```python
from build123d import *

# Parameters (mm, degrees)
EXTRUDE_1_DEPTH       = 245
EXTRUDE_3_DEPTH       = 245
PATTERN_CURVE_1_COUNT = 19
PATTERN_CURVE_1_PITCH = 9.75
SKETCH_3_R            = 2.05
CUT_EXTRUDE_1_DEPTH   = 10
CUT_EXTRUDE_START     = -10
SKETCH_5_R            = 2.05
CUT_EXTRUDE_2_DEPTH   = 10
SKETCH_6_R            = 2.5
CUT_EXTRUDE_3_DEPTH   = 8
SKETCH_7_R            = 2.6
CUT_EXTRUDE_4_DEPTH   = 6
SKETCH_8_R            = 3.4
SKETCH_8_R_2          = 4.5
CUT_EXTRUDE_5_DEPTH   = 6
CUT_EXTRUDE_START_2   = -8
SKETCH_10_R           = 2.5
CUT_EXTRUDE_7_DEPTH   = 8
SKETCH_12_R           = 1.3
SKETCH_12_R_2         = 1.6
SKETCH_12_R_3         = 2.1
CUT_EXTRUDE_8_DEPTH   = 8


with BuildPart() as part:
    # Эскиз1 → Вытянуть1 (new body)
    with BuildSketch(Plane.XY):
        with BuildLine():
            Line((0, 45), (2.564446908, 45))
            ThreePointArc((2.564446908, 45), (3.247630994, 44.730246195), (3.562232066, 44.066519011))
            Line((3.562232066, 44.066519011), (5.5, 15))
            Line((5.5, 15), (194.5, 15))
            Line((194.5, 15), (196.437767934, 44.066519011))
            ThreePointArc((196.437767934, 44.066519011), (196.752369006, 44.730246195), (197.435553092, 45))
            Line((197.435553092, 45), (200, 45))
            Line((200, 45), (200, 0))
            Line((200, 0), (0, 0))
            Line((0, 0), (0, 45))
        make_face()
    extrude(amount=EXTRUDE_1_DEPTH)

    # Эскиз2 → Вытянуть3 (add)
    with BuildSketch(Plane.XY.offset(245)):
        with BuildLine():
            Line((11.5, 44.5), (10, 15))
            Line((10, 15), (14, 15))
            Line((14, 15), (12.5, 44.5))
            ThreePointArc((12.5, 44.5), (12, 45), (11.5, 44.5))
        make_face()
    extrude_3 = extrude(amount=-EXTRUDE_3_DEPTH)

    # Кривая1: Вытянуть3 ×19
    with Locations(*[(i * PATTERN_CURVE_1_PITCH, 0, 0) for i in range(1, PATTERN_CURVE_1_COUNT)]):
        add(extrude_3)

    # Эскиз3 → Вырез-Вытянуть1 (cut)
    with BuildSketch(Plane.XY.offset(245)):
        with Locations((20, 5)):
            Circle(SKETCH_3_R)
        with Locations((100, 5)):
            Circle(SKETCH_3_R)
        with Locations((180, 5)):
            Circle(SKETCH_3_R)
    extrude(amount=-CUT_EXTRUDE_1_DEPTH, mode=Mode.SUBTRACT)

    # Эскиз5 → Вырез-Вытянуть2 (cut)
    with BuildSketch(Plane(origin=(0, 0, 0), x_dir=(-1, 0, 0), z_dir=(0, 0, -1)).offset(CUT_EXTRUDE_START)):
        with Locations(Location((-180, 5, 0), (0, 0, 180))):
            Circle(SKETCH_5_R)
        with Locations(Location((-100, 5, 0), (0, 0, 180))):
            Circle(SKETCH_5_R)
        with Locations(Location((-20, 5, 0), (0, 0, 180))):
            Circle(SKETCH_5_R)
    extrude(amount=CUT_EXTRUDE_2_DEPTH, mode=Mode.SUBTRACT)

    # Эскиз6 → Вырез-Вытянуть3 (cut)
    with BuildSketch(Plane(origin=(0, 0, 0), x_dir=(-1, 0, 0), z_dir=(0, 0, -1))):
        with Locations((-4, 6)):
            Circle(SKETCH_6_R)
        with Locations(Location((-196, 6, 0), (0, 0, 180))):
            Circle(SKETCH_6_R)
    extrude(amount=-CUT_EXTRUDE_3_DEPTH, mode=Mode.SUBTRACT)

    # Эскиз7 → Вырез-Вытянуть4 (cut)
    with BuildSketch(Plane.ZY):
        with Locations(Location((22.5, 20, 0), (0, 0, 270))):
            Circle(SKETCH_7_R)
        with Locations(Location((222.5, 20, 0), (0, 0, 270))):
            Circle(SKETCH_7_R)
        with Locations(Location((122.5, 20, 0), (0, 0, 270))):
            Circle(SKETCH_7_R)
    extrude(amount=-CUT_EXTRUDE_4_DEPTH, mode=Mode.SUBTRACT)

    # Эскиз8 → Вырез-Вытянуть5 (cut)
    with BuildSketch(Plane(origin=(200, 0, 0), x_dir=(0, 0, -1), z_dir=(1, 0, 0))):
        with Locations((-80, 30)):
            Circle(SKETCH_8_R)
        with Locations((-165, 30)):
            Circle(SKETCH_8_R_2)
    extrude(amount=-CUT_EXTRUDE_5_DEPTH, mode=Mode.SUBTRACT)

    # Эскиз10 → Вырез-Вытянуть7 (cut)
    with BuildSketch(Plane.XY.offset(245).offset(CUT_EXTRUDE_START_2)):
        with Locations((196, 6)):
            Circle(SKETCH_10_R)
        with Locations(Location((4, 6, 0), (0, 0, 180))):
            Circle(SKETCH_10_R)
    extrude(amount=CUT_EXTRUDE_7_DEPTH, mode=Mode.SUBTRACT)

    # Эскиз12 → Вырез-Вытянуть8 (cut)
    with BuildSketch(Plane.XZ):
        with Locations((45.75, 202.5)):
            Circle(SKETCH_12_R)
        with Locations((10, 235)):
            Circle(SKETCH_12_R_2)
        with Locations((10, 125)):
            Circle(SKETCH_12_R_2)
        with Locations((160, 235)):
            Circle(SKETCH_12_R_2)
        with Locations((160, 125)):
            Circle(SKETCH_12_R_2)
        with Locations((75, 225)):
            Circle(SKETCH_12_R_3)
        with Locations((100.5, 203)):
            Circle(SKETCH_12_R)
        with Locations((100.5, 158)):
            Circle(SKETCH_12_R)
        with Locations((130, 203)):
            Circle(SKETCH_12_R)
        with Locations((130, 158)):
            Circle(SKETCH_12_R)
    extrude(amount=-CUT_EXTRUDE_8_DEPTH, mode=Mode.SUBTRACT)


solid = part.part
```
For this review, take the finished solid that the model builds, in its own axes (mm). A direction names the side the tool comes from. Round coordinates to 2 decimals unless told otherwise and drop trailing zeros. Use a Markdown table: item, result.
Item 1: Machinability: for faces 1 (the cylindrical face through (198.385, 6.751, 240.944)), 2 (the flat face through (101, 0, 121)), 3 (the flat face through (98.51, 29.96, 124.22)), which of the approach directions +Z, -Z, +X, -X, +Y, -Y give a long, thin tool a straight path to every point of the face, cutting with its end or side? Answer none if there is none.
Resolved:
| item | result |
|---|---|
| face 1 | +Z |
| face 2 | +Z, -Z, +X, -X, -Y |
| face 3 | +Z, -Z, +Y |
Item 2: For line 1 along Z through (x, y) = (160, 2); line 2 along Z through (x, y) = (3.5, 20); line 3 along X through (y, z) = (3, 202), list the stretches that pass through material, from the lowest coordinate up. Write a range as [from, to].
Resolved:
| item | result |
|---|---|
| line 1 | z = [0, 123.4], [126.6, 233.4], [236.6, 245] |
| line 2 | z = [0, 19.9], [25.1, 119.9], [125.1, 219.9], [225.1, 245] |
| line 3 | x = [0, 44.55], [46.95, 99.67], [101.33, 129.17], [130.83, 200] |
Item 3: Draft analysis for pull direction Z (two halves, no side actions). For faces 4 (the flat face through (101, 18, 0)), 5 (the cylindrical face through (2.63, 17.52, 23.28)), 6 (the cylindrical face through (1.615, 5.249, 240.944)), state which applies: +Z half, -Z half, draft (parallel to the pull), parting line (faces both ways), or undercut.
Resolved:
| item | result |
|---|---|
| face 4 | -Z half |
| face 5 | undercut |
| face 6 | draft |
Item 4: For pin 1 (3 mm diameter, centred on x = 25.5, z = 98.5, fed in from +Y); pin 2 (2.5 mm diameter, centred on x = 4, y = 7, fed in from +Z); pin 3 (6.5 mm diameter, centred on x = 35, z = 177, fed in from +Y), all flat-tipped, find the tip position at first contact; note any pin that passes through.
Resolved:
| item | result |
|---|---|
| pin 1 | stops at y = 15 |
| pin 2 | stops at z = 237 |
| pin 3 | stops at y = 44.93 |
